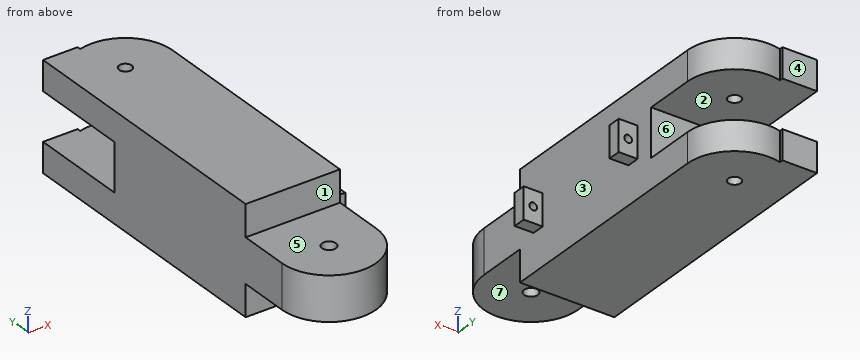
from build123d import *

# Parameters (mm, degrees)
LINK1_BODY_DEPTH       = 8.5
TONGUE_CUT_DEPTH       = 56.258483512
TONGUE_CUT_DEPTH_BACK  = 56.258483512
SKETCH1_W              = 5.5
SKETCH1_H              = 15.998130079
SKETCH7_W              = 5.5
SKETCH7_H              = 7.8
BOSS_EXTRUDE1_DEPTH    = 8.5
SLOT_CUT_DEPTH         = 55.003148056
SLOT_CUT_DEPTH_BACK    = 55.003148056
SKETCH2_W              = 7.6
SKETCH2_H              = 18
PIN_HOLES_DEPTH        = 55.003148056
PIN_HOLES_DEPTH_BACK   = 55.003148056
SKETCH3_R              = 1.1
SKETCH3_R_2            = 1
SKETCH4_W              = 3.5
SKETCH4_H              = 2
GUIDE_BLOCK_1_DEPTH    = 2.5
SKETCH5_W              = 3.5
SKETCH5_H              = 2
GUIDE_BLOCK_2_DEPTH    = 2.5
CORD_GUIDES_DEPTH      = 55.500938464
CORD_GUIDES_DEPTH_BACK = 55.500938464
SKETCH6_R              = 0.6


with BuildPart() as part:
    # Link1_Outline → Link1_Body (new, symmetric)
    with BuildSketch(Plane.XY):
        with BuildLine():
            Line((-7.5, 0), (-7.5, 45))
            ThreePointArc((-7.5, 45), (0, 52.5), (7.5, 45))
            Line((7.5, 45), (7.5, 0))
            ThreePointArc((7.5, 0), (0, -7.5), (-7.5, 0))
        make_face()
    extrude(amount=LINK1_BODY_DEPTH, both=True)

    # Sketch1 → Tongue_Cut (cut, two sides: drawn at the far end of the back side and taken through both)
    with BuildSketch(Plane(origin=(7.5, 0, 0), x_dir=(0, 0, -1), z_dir=(1, 0, 0)).offset(-TONGUE_CUT_DEPTH_BACK)):
        with Locations((6.25, -0.00093496)):
            Rectangle(SKETCH1_W, SKETCH1_H)
        with Locations((-6.25, -0.00093496)):
            Rectangle(SKETCH1_W, SKETCH1_H)
    extrude(amount=TONGUE_CUT_DEPTH + TONGUE_CUT_DEPTH_BACK, mode=Mode.SUBTRACT)

    # Sketch7 → Boss-Extrude1 (add, symmetric)
    with BuildSketch(Plane.XY):
        with Locations((-4.75, 48.9)):
            Rectangle(SKETCH7_W, SKETCH7_H)
    extrude(amount=BOSS_EXTRUDE1_DEPTH, both=True)

    # Sketch2 → Slot_Cut (cut, two sides: drawn at the far end of the back side and taken through both)
    with BuildSketch(Plane(origin=(0, 0, 0), x_dir=(0, 0, -1), z_dir=(1, 0, 0)).offset(-SLOT_CUT_DEPTH_BACK)):
        with Locations((0, 46)):
            Rectangle(SKETCH2_W, SKETCH2_H)
    extrude(amount=SLOT_CUT_DEPTH + SLOT_CUT_DEPTH_BACK, mode=Mode.SUBTRACT)

    # Sketch3 → Pin_Holes (cut, two sides: drawn at the far end of the back side and taken through both)
    with BuildSketch(Plane.XY.offset(-PIN_HOLES_DEPTH_BACK)):
        Circle(SKETCH3_R)
        with Locations((0, 45)):
            Circle(SKETCH3_R_2)
    extrude(amount=PIN_HOLES_DEPTH + PIN_HOLES_DEPTH_BACK, mode=Mode.SUBTRACT)

    # Sketch4 → Guide_Block_1 (add, symmetric)
    with BuildSketch(Plane.XY):
        with Locations((8.75, 12)):
            Rectangle(SKETCH4_W, SKETCH4_H)
    extrude(amount=GUIDE_BLOCK_1_DEPTH, both=True)

    # Sketch5 → Guide_Block_2 (add, symmetric)
    with BuildSketch(Plane.XY):
        with Locations((8.750585387, 33)):
            Rectangle(SKETCH5_W, SKETCH5_H)
    extrude(amount=GUIDE_BLOCK_2_DEPTH, both=True)

    # Sketch6 → Cord_Guides (cut, two sides: drawn at the far end of the back side and taken through both)
    with BuildSketch(Plane(origin=(0, 0, 0), x_dir=(1, 0, 0), z_dir=(0, 1, 0)).offset(-CORD_GUIDES_DEPTH_BACK)):
        with Locations(Location((9, 0, 0), (0, 0, 90))):
            Circle(SKETCH6_R)
    extrude(amount=CORD_GUIDES_DEPTH + CORD_GUIDES_DEPTH_BACK, mode=Mode.SUBTRACT)


solid = part.part
Geometry: final body of the model. Coordinates: model frame, mm. Face numbers are marked on the shaded views. A direction names the side the tool comes from. Give positions to 0.01 mm unless a question says otherwise; leave off trailing zeros. Loops run counter-clockwise (first coordinate to the right, second up) from the corner with the lowest first, then second, coordinate; pieces in that order, holes last. Notation, with made-up numbers: M 81,13.5 L 90,13.5 A33 cw 90,46.5 Z; hole C -26.75,20 d3. An arc over 180 degrees is marked long. Put each result on its own line as item: value. Start each with the question number.
1) Cut plane B-B (y = 12). Output: boundary loops of the cut face in (x, z), then the cut area to 3 significant figures.
2) Pull-direction query (Y, two-part tool) for the marked faces 1, 2 and 3; classes: pulls with the +Y half, pulls with the -Y half, needs draft (parallel to the pull), parting line crosses it, or undercut.
3) Cut plane A-A (z = 0). Output: boundary loops of the cut face in (x, y), then the cut area to 3 significant figures.
4) Contact query for flat-ended pins moving along their axis: pin 1 (8 mm diameter, centred on x = -5.5, z = -2.5, fed in from -Y); pin 2 (1.5 mm diameter, centred on x = -5.5, z = 1, fed in from +Y); pin 3 (1.4 mm diameter, centred on x = 9, z = 0, fed in from -Y). Output: stop coordinate, or through.
5) Access query for the marked faces 4, 5, 6 and 7. Directions: +Z, -Z, +X, -X, +Y, -Y. A direction counts if a zero-diameter tool reaches every point of the face in a straight line with its end or side. Return the directions, or none.
6) Cut plane C-C (x = 9). Output: boundary loops of the cut face in (y, z).
7) Ray query, line 1 along Y through (x, z) = (0, -1); line 2 along Y through (x, z) = (0, -7.25); line 3 along X through (y, z) = (33.2, 0). Return the intervals inside material, ascending.
8) Cut plane D-D (z = 7.25). Output: boundary loops of the cut face in (x, y), then the cut area to 3 significant figures.
Verdict:
1. outline: M -7.5,-8.5 L 7.5,-8.5 L 7.5,-2.5 L 10.5,-2.5 L 10.5,2.5 L 7.5,2.5 L 7.5,8.5 L -7.5,8.5 Z; hole C 9,0 d1.2
1. area: 269 mm2
2. face 1: pulls with the -Y half
2. face 2: needs draft
2. face 3: undercut
3. outline: M -7.5,0 A7.5 ccw 7.5,0 L 7.5,11 L 8.4,11 L 8.4,13 L 7.5,13 L 7.5,32 L 8.4,32 L 8.4,34 L 7.5,34 L 7.5,37 L -7.5,37 Z; M 9.6,11 L 10.5,11 L 10.5,13 L 9.6,13 Z; M 9.6,32 L 10.5,32 L 10.5,34 L 9.6,34 Z; hole C 0,0 d2.2
3. area: 647 mm2
4. pin 1: y = -7.35
4. pin 2: y = 37
4. pin 3: y = 11
5. face 4: +Z, -Z, +X, -X, +Y
5. face 5: +Z, +X, -X, -Y
5. face 6: +X, -X, +Y
5. face 7: -Z, +X, -X, -Y
6. outline: M 11,-2.5 L 13,-2.5 L 13,-0.6 L 11,-0.6 Z; M 11,0.6 L 13,0.6 L 13,2.5 L 11,2.5 Z; M 32,-2.5 L 34,-2.5 L 34,-0.6 L 32,-0.6 Z; M 32,0.6 L 34,0.6 L 34,2.5 L 32,2.5 Z
7. line 1: -7.5 to -1.1, 1.1 to 37
7. line 2: 8 to 44, 46 to 52.5
7. line 3: -7.5 to 8.4, 9.6 to 10.5
8. outline: M -7.5,8 L 7.5,8 L 7.5,45 A7.5 ccw -2,52.23 L -2,52.8 L -7.5,52.8 Z; hole C 0,45 d2
8. area: 654 mm2
